Input: dimensioned drawing with shaded views. Units: mm. Origin: part minimum x, y, z. A direction names the side the tool comes from. Give positions to 0.01 mm unless a question says otherwise; leave off trailing zeros. Order: outer loops, then holes, each group sorted by start corner. A loop starts at its lowest first (then second) coordinate and runs counter-clockwise, first axis right, second up. Notation, with made-up numbers: (61, 66) - (65, 66) arc R15 ccw to (65, 75) - close; hole circle Ø3 at (61.5, -35). An arc over 180 degrees is marked (long way). Use a Markdown table: item, result.
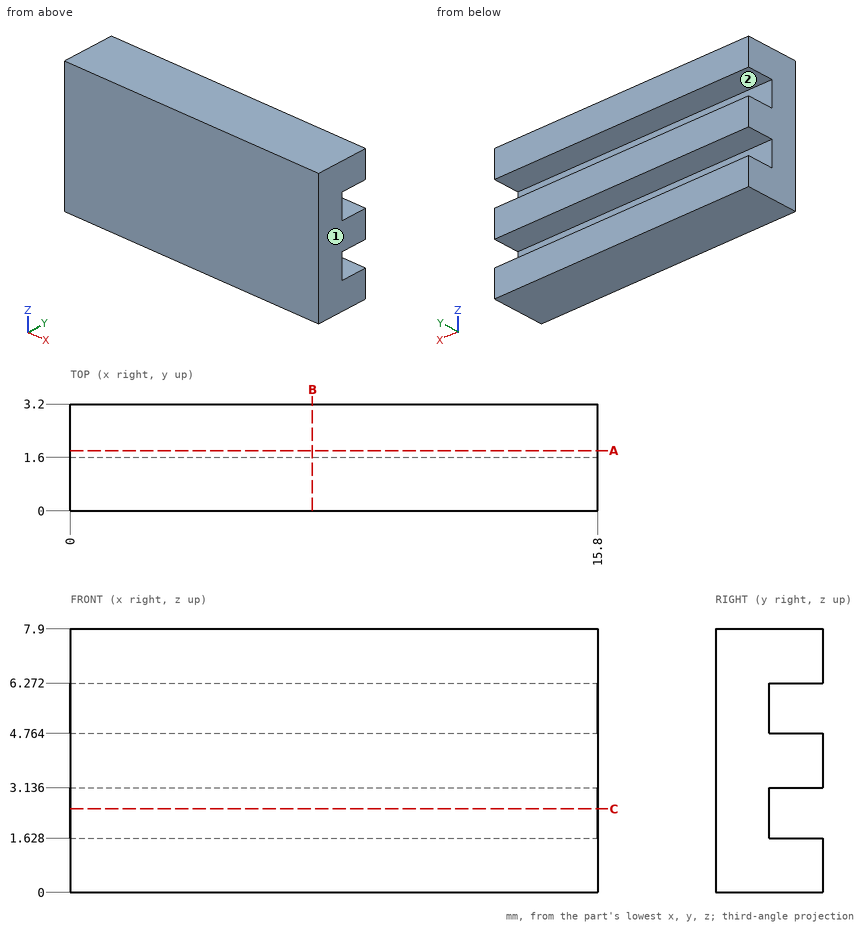
1. Material intervals for line 1 along Z through (x, y) = (8, 2.6); line 2 along Y through (x, z) = (2.25, 2), sorted ascending.
Response:
| item | result |
|---|---|
| line 1 | z = 0 to 1.63, 3.14 to 4.76, 6.27 to 7.9 |
| line 2 | y = 0 to 1.6 |
2. Section query C-C (z = 2.5). Return loops of the section in (x, y).
Response:
| item | result |
|---|---|
| outline | (0, 0) - (15.8, 0) - (15.8, 1.6) - (0, 1.6) - close |
3. Pin query (flat end, axial travel): pin 1 (0.8 mm diameter, centred on x = 7.5, z = 5.5, fed in from +Y). Return the tip coordinate at first contact, or that it passes through.
Response:
| item | result |
|---|---|
| pin 1 | stops at y = 1.6 |
4. Section query B-B (x = 7.25). Return loops of the section in (y, z).
Response:
| item | result |
|---|---|
| outline | (0, 0) - (3.2, 0) - (3.2, 1.63) - (1.6, 1.63) - (1.6, 3.14) - (3.2, 3.14) - (3.2, 4.76) - (1.6, 4.76) - (1.6, 6.27) - (3.2, 6.27) - (3.2, 7.9) - (0, 7.9) - close |
5. Section query A-A (y = 1.8). Return loops of the section in (x, z).
Response:
| item | result |
|---|---|
| outline | (0, 0) - (15.8, 0) - (15.8, 1.63) - (0, 1.63) - close; (0, 3.14) - (15.8, 3.14) - (15.8, 4.76) - (0, 4.76) - close; (0, 6.27) - (15.8, 6.27) - (15.8, 7.9) - (0, 7.9) - close |
6. Set-up query: the marked faces 1 and 2. Return all of +Z, -Z, +X, -X, +Y, -Y with unobstructed straight access to the full face (end or side cutting, diameter ignored); none if empty.
Response:
| item | result |
|---|---|
| face 1 | +Z, -Z, +X, +Y, -Y |
| face 2 | +X, -X, +Y |
